Geometry: final body of the model. Coordinates: model frame, mm. Face numbers are marked on the shaded views. A direction names the side the tool comes from. Coordinates: 2 decimals unless noted, no trailing zeros. Loops run counter-clockwise (first coordinate to the right, second up) from the corner with the lowest first, then second, coordinate; pieces in that order, holes last. Notation, with made-up numbers: (-3, 83.25) - (44, 83.25) arc R15 cw to (44, 94.25) - close; hole circle Ø7 at (62.5, 72). An arc over 180 degrees is marked (long way). Put each result on its own line as item: value. Start each with the question number.
1) Section D-D on z = 35. Output: boundary loops of the cut face in (x, y).
2) Material intervals for line 1 along Z through (x, y) = (35, 1.25); line 2 along Z through (x, y) = (53.5, 2.4); line 3 along X through (y, z) = (1.2, 65), sorted ascending. Write a range as from..to.
3) Section B-B on z = 65. Output: boundary loops of the cut face in (x, y).
4) Reachability of the marked faces 1, 2 and 3 from +Z, -Z, +X, -X, +Y, -Y: full face, straight path, thin tool, end or side. Return the list, or none.
5) Section C-C on x = 60. Output: boundary loops of the cut face in (y, z).
6) Contact query for flat-ended pins moving along their axis: pin 1 Ø0.6 at (x, y) = (110.5, 0.5) entering from -Z; pin 2 Ø4 at (x, z) = (8, 35) entering from +Y; pin 3 Ø1.5 at (y, z) = (2, 64.5) entering from -X. Output: stop coordinate, or through.
7) Section A-A on x = 42. Output: boundary loops of the cut face in (y, z), and give its area (3 significant figures).
Autodesk Fusion 360 part; units mm, degrees
sketch "Sketch1" plane through (0, 0, 0) normal (0, 1, 0) x (1, 0, 0)
  circle A0 centre (18.4015, -12.4035) radius 2
  line L0 (-11, -35) -> (125, -35)
  line L1 (60, 10) -> (60, -83.0941)
  circle A1 centre (101.5985, -12.4035) radius 2
  circle A2 centre (18.4015, -57.5965) radius 2
  circle A3 centre (101.5985, -57.5965) radius 2
  line L2 (5, -45) -> (13, -45)
  line L3 (13, -45) -> (13, -25)
  line L4 (13, -25) -> (5, -25)
  line L5 (3, -27) -> (3, -43)
  circle A4 centre (8, -35) radius 1.5
  line L6 (97, -50) -> (23, -50)
  line L7 (20, -47) -> (20, -23)
  line L8 (23, -20) -> (97, -20)
  line L9 (100, -23) -> (100, -47)
  arc A5 (20, -47) -> (23, -50) centre (23, -47) ccw
  arc A6 (23, -20) -> (20, -23) centre (23, -23) ccw
  arc A7 (97, -50) -> (100, -47) centre (97, -47) ccw
  arc A8 (100, -23) -> (97, -20) centre (97, -23) ccw
  arc A9 (3, -43) -> (5, -45) centre (5, -43) ccw
  arc A10 (5, -25) -> (3, -27) centre (5, -27) ccw
  line L10 (106, -45) -> (114, -45)
  line L11 (116, -43) -> (116, -27)
  line L12 (114, -25) -> (106, -25)
  line L13 (106, -25) -> (106, -45)
  arc A11 (114, -45) -> (116, -43) centre (114, -43) ccw
  arc A12 (116, -27) -> (114, -25) centre (114, -27) ccw
  circle A13 centre (111, -35) radius 1.5
  line L14 (92.023, -6.7335) -> (99.623, -6.7335)
  line L15 (99.623, -6.7335) -> (99.623, -1.1335)
  line L16 (99.623, -1.1335) -> (92.023, -1.1335)
  line L17 (92.023, -1.1335) -> (92.023, -6.7335)
  circle A14 centre (35, -65) radius 2.25
  line L18 (53, -62) -> (67.6, -62)
  line L19 (67.6, -62) -> (67.6, -67.9)
  line L20 (67.6, -67.9) -> (53, -67.9)
  line L21 (53, -67.9) -> (53, -62)
  line L22 (13, -1) -> (13, -69)
  line L23 (16, -72) -> (103, -72)
  line L24 (106, -69) -> (106, -1)
  line L25 (103, 2) -> (16, 2)
  arc A15 (16, 2) -> (13, -1) centre (16, -1) ccw
  arc A16 (106, -1) -> (103, 2) centre (103, -1) ccw
  arc A17 (13, -69) -> (16, -72) centre (16, -69) ccw
  arc A18 (103, -72) -> (106, -69) centre (103, -69) ccw
  point P0 (0, -70)
  point P1 (3, -45)
  point P2 (116, -45)
  point P3 (109, -75)
  dimension "d8" = 4
  dimension "d11" = 10
  dimension "d12" = 3
  dimension "d17" = 3
  dimension "d18" = 3
  dimension "d19" = 3
  dimension "d20" = 3
  dimension "d21" = 2
  dimension "d22" = 2
  dimension "d33" = 10
  dimension "d34" = 2
  dimension "d35" = 2
  dimension "d36" = 3
  dimension "d51" = 7.6
  dimension "d52" = 5.6
  dimension "d53" = 4.5
  dimension "d54" = 5.9
  dimension "d55" = 14.6
  dimension "d63" = 3
  dimension "d64" = 3
  dimension "d65" = 3
  dimension "d66" = 3
extrude "Extrude10" add sketch "Sketch1" along normal blind 3 contours L0 L1 L3 L7 L8 A6 L22 L25 A15 | L0 L1 L3 L6 L7 A5 L18 L20 L21 L22 L23 A17 | L0 L1 L8 L9 A8 L13 L24 L25 A16 | L0 L1 L6 L9 A7 L13 L18 L19 L20 L23 L24 A18
extrude "Extrude11" add sketch "Sketch1" along normal blind 2 contours L0 L3 L4 L5 A4 A10 L22 | L0 L2 L3 L5 A4 A9 L22 | L0 L11 L12 L13 A12 A13 L24 | L0 L10 L11 L13 A11 A13 L24
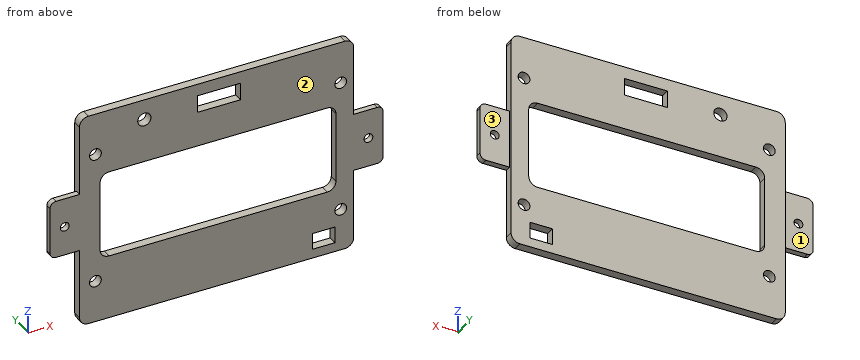
Answer block:
1. outline: (3, 0) - (6.5, 0) - (6.5, 2) - (3, 2) - close; (9.5, 0) - (20, 0) - (20, 3) - (13, 3) - (13, 2) - (9.5, 2) - close; (100, 0) - (109.5, 0) - (109.5, 2) - (106, 2) - (106, 3) - (100, 3) - close; (112.5, 0) - (116, 0) - (116, 2) - (112.5, 2) - close
2. line 1: z = -2..20, 50..62.75, 67.25..72
2. line 2: z = -2..20, 50..62, 67.9..72
2. line 3: x = 13..32.75, 37.25..53, 67.6..106
3. outline: (13, 0) - (32.75, 0) - (32.75, 3) - (13, 3) - close; (37.25, 0) - (53, 0) - (53, 3) - (37.25, 3) - close; (67.6, 0) - (106, 0) - (106, 3) - (67.6, 3) - close
4. face 1: +Z, -Z, -X, +Y
4. face 2: +Z, -Z, +X, -X, -Y
4. face 3: +Z, -Z, +X, +Y
5. outline: (0, -2) - (3, -2) - (3, 20) - (0, 20) - close; (0, 50) - (3, 50) - (3, 62) - (0, 62) - close; (0, 67.9) - (3, 67.9) - (3, 72) - (0, 72) - close
6. pin 1: stops at z = 25
6. pin 2: stops at y = 2
6. pin 3: stops at x = 13
7. outline: (0, -2) - (3, -2) - (3, 20) - (0, 20) - close; (0, 50) - (3, 50) - (3, 72) - (0, 72) - close
7. area: 132 mm²
